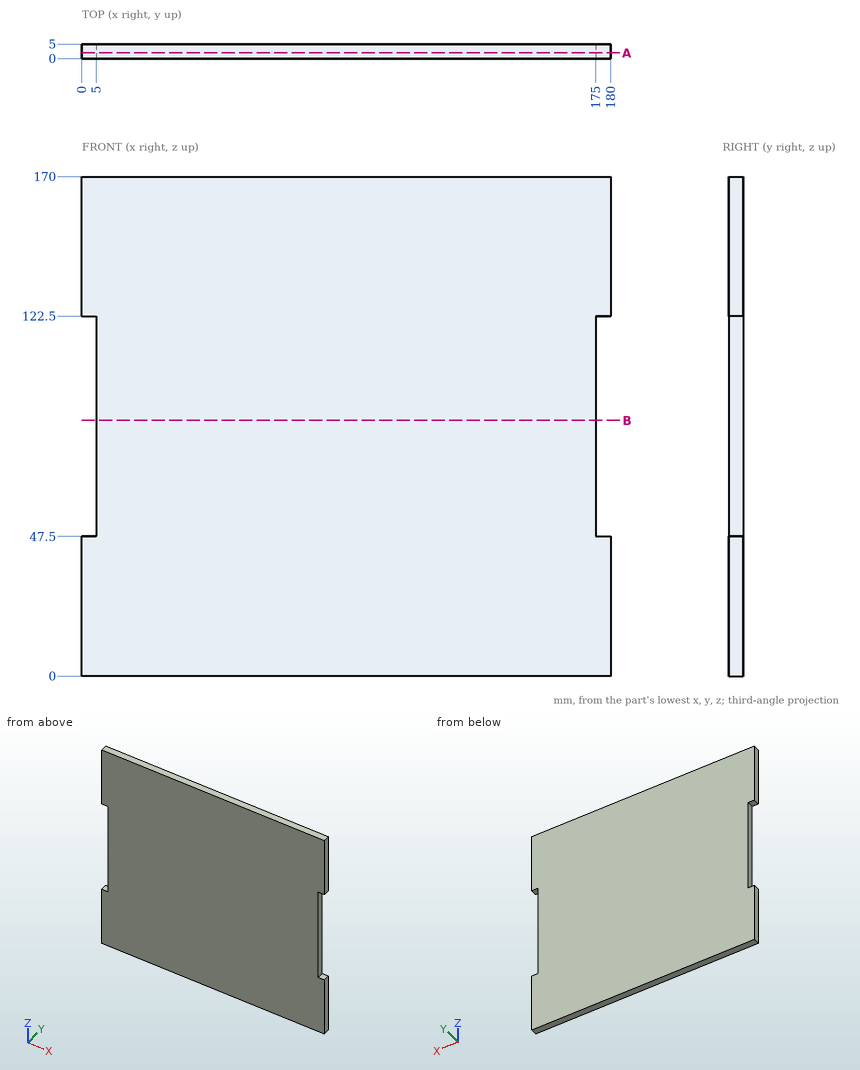
Here's the drawing with two shaded views (mm, measured from the low corner). I have some questions. Coordinates: 2 decimals unless noted, no trailing zeros. Order: outer loops, then holes, each group sorted by start corner. A loop starts at its lowest first (then second) coordinate and runs counter-clockwise, first axis right, second up.
Item 1: If we section it at A-A on y = 2: List the corners of the cut face in (x, z) for me, plus the area to 4 significant figures.
Result sheet:
outline: (0, 0) - (180, 0) - (180, 47.5) - (175, 47.5) - (175, 122.5) - (180, 122.5) - (180, 170) - (0, 170) - (0, 122.5) - (5, 122.5) - (5, 47.5) - (0, 47.5) - close
area: 29,850 mm2
Item 2: If we section it at B-B on z = 87: List the corners of the cut face in (x, y) for me.
Result sheet:
outline: (5, 0) - (175, 0) - (175, 5) - (5, 5) - close
Item 3: I need wall thicknesses on line 1 (X direction, y = 4.65, z = 114). Which ranges of the line are inside material? Lowest first, please.
Result sheet:
line 1: x = 5 to 175
Item 4: For P1, Ø2.5, axis at y = 2.5, z = 70, coming from the +X side, with a flat end and sliding along its axis, tell me the tip position at first contact or that it passes through.
Result sheet:
P1: stops at x = 175
